Design review of the part shown in the three views and the two pictorial views. Dimensions are in mm from the part's minimum x, y and z. Give positions to 0.01 mm unless a question says otherwise; leave off trailing zeros. Order: outer loops, then holes, each group sorted by start corner. A loop starts at its lowest first (then second) coordinate and runs counter-clockwise, first axis right, second up. Notation, with made-up numbers: M 61,17.25 L 83,17.25 A18 cw 83,28.25 Z; hole C -19,67 d1. An arc over 180 degrees is marked long. Answer as a JSON object with one key per item and string values.
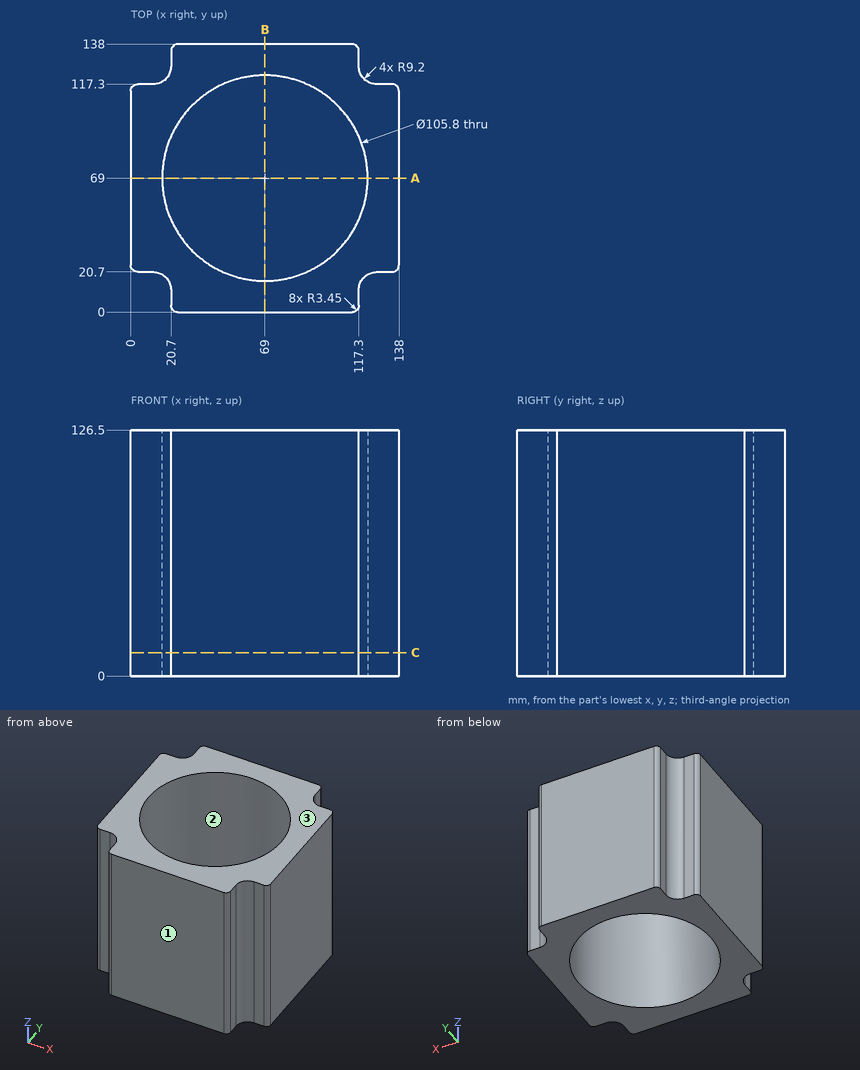
(1) We need section C-C (z = 12). Write out the cut boundary in (x, y).
Checked values:
{"outline": "M 0,24.15 A3.45 ccw 3.45,20.7 L 11.5,20.7 A9.2 cw 20.7,11.5 L 20.7,3.45 A3.45 ccw 24.15,0 L 113.85,0 A3.45 ccw 117.3,3.45 L 117.3,11.5 A9.2 cw 126.5,20.7 L 134.55,20.7 A3.45 ccw 138,24.15 L 138,113.85 A3.45 ccw 134.55,117.3 L 126.5,117.3 A9.2 cw 117.3,126.5 L 117.3,134.55 A3.45 ccw 113.85,138 L 24.15,138 A3.45 ccw 20.7,134.55 L 20.7,126.5 A9.2 cw 11.5,117.3 L 3.45,117.3 A3.45 ccw 0,113.85 Z; hole C 69,69 d105.8"}
(2) To check wall thickness, follow L1, parallel to Y at x = 69, z = 82; L2, parallel to X at y = 109, z = 100; L3, parallel to X at y = 45, z = 80.5. State the ranges of each line that lie inside material, in increasing order. Write a range as from..to.
Checked values:
{"L1": "y = 0..16.1, 121.9..138", "L2": "x = 0..34.38, 103.62..138", "L3": "x = 0..21.86, 116.14..138"}
(3) Insertion check: pin 1 (2.5 mm diameter, centred on x = 130, z = 56.5, fed in from -Y); pin 2 (2.5 mm diameter, centred on x = 131, z = 93.5, fed in from +Y); pin 3 (6.5 mm diameter, centred on y = 6.5, z = 32, fed in from -X). Each pin has a flat end and moves straight along its axis. Give the tip position at first contact, or say it passes through.
Checked values:
{"pin 1": "stops at y = 20.7", "pin 2": "stops at y = 117.3", "pin 3": "stops at x = 20.7"}
(4) We need section A-A (y = 69). Write out the cut boundary in (x, z).
Checked values:
{"outline": "M 0,0 L 16.1,0 L 16.1,126.5 L 0,126.5 Z; M 121.9,0 L 138,0 L 138,126.5 L 121.9,126.5 Z"}
(5) Draft analysis for pull direction Y (two halves, no side actions). For the marked faces 1, 2 and 3, state which applies: +Y half, -Y half, draft (parallel to the pull), parting line (faces both ways), or undercut.
Checked values:
{"face 1": "-Y half", "face 2": "undercut", "face 3": "draft"}
